Autodesk Fusion 360 part; units mm, degrees
sketch "Sketch1" plane through (0, 0, 0) normal (0, 1, 0) x (1, 0, 0)
  line L0 (0, 0) -> (5.5, 0)
  line L1 (0, -3.5) -> (2.625, -3.5)
  line L2 (2.625, -3.5) -> (5.5, 0)
  line L3 (0, -1.75) -> (0, -22.5)
  line L4 (0, -3.5) -> (-2.625, -3.5)
  line L5 (-2.625, -3.5) -> (-5.5, 0)
  line L6 (0, 0) -> (-5.5, 0)
  dimension "d1" = 5.5
  dimension "d2" = 2.625
  dimension "d3" = 3.5
extrude "Extrude1" add sketch "Sketch1" along normal blind 38
sketch "Sketch2" plane through (0, 0, 3.5) normal (0, 0, 1) x (-1, 0, 0)
  line L0 (2.625, 0) -> (-2.625, 0)
  line L1 (-2.625, 0) -> (-2.625, -38)
  line L2 (-2.625, -38) -> (2.625, -38)
  line L3 (2.625, -38) -> (2.625, 0)
  line L4 (0, -38) -> (0, 0) construction
  line L5 (2.72, -29.9296) -> (0, -28.3592)
  line L6 (0, -28.3592) -> (-2.72, -29.9296)
  line L7 (-2.72, -29.9296) -> (-2.72, -33.0704)
  line L8 (-2.72, -33.0704) -> (0, -34.6408)
  line L9 (0, -34.6408) -> (2.72, -33.0704)
  line L10 (2.72, -33.0704) -> (2.72, -29.9296)
  line L11 (2.72, -4.9296) -> (0, -3.3592)
  line L12 (0, -3.3592) -> (-2.72, -4.9296)
  line L13 (-2.72, -4.9296) -> (-2.72, -8.0704)
  line L14 (-2.72, -8.0704) -> (0, -9.6408)
  line L15 (0, -9.6408) -> (2.72, -8.0704)
  line L16 (2.72, -8.0704) -> (2.72, -4.9296)
  point P0 (0, -31.5)
  point P1 (0, -6.5)
  dimension "d6" = 2.72
  dimension "d7" = 2.72
  dimension "d8" = 25
  dimension "d9" = 6.5
extrude "Extrude2" cut sketch "Sketch2" against normal blind 2.2 contours L1 L3 L11 L12 L14 L15 | L1 L3 L5 L6 L8 L9
hole "Hole1" at (0, 31.5, 3.5) at (0, 6.5, 3.5) direction (0, 0, -1) diameter 3.4 depth 16 tip angle 118
equation "d2 = ( 5.25 / 2 ) * 1 mm"
equation "d6 = ( 5.44 / 2 ) * 1 mm"
equation "d7 = ( 5.44 / 2 ) * 1 mm"
Verification items for the finished model (mm, model axes). A direction names the side the tool comes from. Coordinates: 2 decimals unless noted, no trailing zeros. Write each loop counter-clockwise with the first axis right and the second up, starting at its lowest first coordinate (ties: lowest second). Pieces come first, ordered by that corner, then holes. Notation, with made-up numbers: M -40,30.5 L -3,30.5 A6 cw -3,38.5 Z; hole C 85.5,39.5 d7. An arc over 180 degrees is marked long. One line per item, written item: value.
Item 1: Section check C-C, the plane y = 22. Record the boundary of the cut face in (x, z) (3 decimals).
Check sheet entries:
outline: M -5.5,0 L 5.5,0 L 2.625,3.5 L -2.625,3.5 Z
Item 2: Scan lines: line 1 along Y through (x, z) = (0, 0.9); line 2 along Y through (x, z) = (-1.25, 1.95); line 3 along X through (y, z) = (34.5, 3.2). Record each from-to range of solid material in increasing order.
Check sheet entries:
line 1: y = 0 to 4.8, 8.2 to 29.8, 33.2 to 38
line 2: y = 0 to 4.08, 8.92 to 29.08, 33.92 to 38
line 3: x = -2.87 to -0.24, 0.24 to 2.87
Item 3: Gauge pin test, flat ends, axial feed: pin 1 Ø2 at (y, z) = (23.5, 0.5) entering from +X; pin 2 Ø1.1 at (y, z) = (31, 2) entering from -X; pin 3 Ø2 at (y, z) = (31, 0.5) entering from -X. Record the tip position at first contact, or that the pin passes through.
Check sheet entries:
pin 1: stops at x = 5.5
pin 2: stops at x = -4.31
pin 3: stops at x = -5.5
Item 4: Section check A-A, the plane y = 31.5. Record the boundary of the cut face in (x, z) (3 decimals), plus the area to 3 significant figures.
Check sheet entries:
outline: M -5.5,0 L -1.7,0 L -1.7,1.3 L -2.625,1.3 L -2.625,3.5 Z; M 1.7,0 L 5.5,0 L 2.625,3.5 L 2.625,1.3 L 1.7,1.3 Z
area: 12.5 mm^2
Item 5: Access from +Z, -Z, +X, -X, +Y, -Y to the whole of each face (thin tool, end or side, straight path). Record for faces 5 (the flat face through (1.331, 33.872, 2.415)), 6 (the cylindrical face through (0.65, 29.93, 0.64)).
Check sheet entries:
face 5: +Z
face 6: +Z, -Z
Item 6: Mould release check, pull along X, two halves, no side actions. Record for faces 1 (the flat face through (-2.625, 7, 2)), 2 (the flat face through (0, 19, 0)), 3 (the flat face through (2.625, 6, 2)), 4 (the flat face through (4.042, 18.734, 1.774)): pulls with the +X half, pulls with the -X half, needs draft (parallel to the pull), parting line crosses it, or undercut.
Check sheet entries:
face 1: undercut
face 2: needs draft
face 3: undercut
face 4: pulls with the +X half
Item 7: Section check D-D, the plane x = -4. Record the boundary of the cut face in (y, z).
Check sheet entries:
outline: M 0,0 L 38,0 L 38,1.83 L 0,1.83 Z
Item 8: Section check B-B, the plane x = -0.75. Record the boundary of the cut face in (y, z).
Check sheet entries:
outline: M 0,0 L 4.97,0 L 4.97,1.3 L 3.79,1.3 L 3.79,3.5 L 0,3.5 Z; M 8.03,0 L 29.97,0 L 29.97,1.3 L 28.79,1.3 L 28.79,3.5 L 9.21,3.5 L 9.21,1.3 L 8.03,1.3 Z; M 33.03,0 L 38,0 L 38,3.5 L 34.21,3.5 L 34.21,1.3 L 33.03,1.3 Z
